The listing builds one solid part. Answer for the finished solid, in the listing's coordinates (mm). A direction names the side the tool comes from. Give positions to 0.01 mm unless a question says otherwise; leave off trailing zeros. Order: outer loops, then holes, each group sorted by start corner. A loop starts at its lowest first (then second) coordinate and runs counter-clockwise, first axis right, second up. Notation, with made-up numbers: (2, 46.5) - (41, 46.5) arc R19 cw to (41, 77.5) - close; hole circle Ø11 at (-37.75, 9.25). An arc over 180 degrees is marked (long way). Answer in a Markdown table with one row per item.
from build123d import *

# Parameters (mm, degrees)
AUFSATZ_LINEAR_AUSTRAGEN1_DEPTH = 5


with BuildPart() as part:
    # Skizze1 → Aufsatz-Linear austragen1 (new body)
    with BuildSketch(Plane.XY):
        Polygon((460.89618142, 291.663856447), (470.89618142, 291.663856447), (470.89618142, 296.663856447), (480.89618142, 296.663856447), (480.89618142, 291.663856447), (490.89618142, 291.663856447), (490.89618142, 296.663856447), (500.89618142, 296.663856447), (500.89618142, 291.663856447), (510.89618142, 291.663856447), (510.89618142, 296.663856447), (520.89618142, 296.663856447), (520.89618142, 291.663856447), (530.89618142, 291.663856447), (530.89618142, 296.663856447), (540.89618142, 296.663856447), (540.89618142, 291.663856447), (550.89618142, 291.663856447), (550.89618142, 296.663856447), (560.89618142, 296.663856447), (560.89618142, 291.663856447), (570.89618142, 291.663856447), (570.89618142, 296.663856447), (580.89618142, 296.663856447), (580.89618142, 291.663856447), (590.89618142, 291.663856447), (590.89618142, 296.663856447), (600.89618142, 296.663856447), (600.89618142, 291.663856447), (610.89618142, 291.663856447), (610.89618142, 296.663856447), (620.89618142, 296.663856447), (620.89618142, 291.663856447), (630.89618142, 291.663856447), (630.89618142, 296.663856447), (640.89618142, 296.663856447), (640.89618142, 291.663856447), (650.89618142, 291.663856447), (680.89618142, 261.663856447), (685.89618142, 261.663856447), (685.89618142, 251.663856447), (680.89618142, 251.663856447), (680.89618142, 241.663856447), (685.89618142, 241.663856447), (685.89618142, 231.663856447), (680.89618142, 231.663856447), (680.89618142, 221.663856447), (685.89618142, 221.663856447), (685.89618142, 211.663856447), (680.89618142, 211.663856447), (680.89618142, 201.663856447), (685.89618142, 201.663856447), (685.89618142, 191.663856447), (680.89618142, 191.663856447), (680.89618142, 181.663856447), (685.89618142, 181.663856447), (685.89618142, 171.663856447), (680.89618142, 171.663856447), (680.89618142, 161.663856447), (685.89618142, 161.663856447), (685.89618142, 151.663856447), (680.89618142, 151.663856447), (680.89618142, 141.663856447), (685.89618142, 141.663856447), (685.89618142, 131.663856447), (680.89618142, 131.663856447), (680.89618142, 121.663856447), (685.89618142, 121.663856447), (685.89618142, 111.663856447), (680.89618142, 111.663856447), (680.89618142, 101.663856447), (685.89618142, 101.663856447), (685.89618142, 91.663856447), (680.89618142, 91.663856447), (680.89618142, 81.663856447), (685.89618142, 81.663856447), (685.89618142, 71.663856447), (680.89618142, 71.663856447), (680.89618142, 61.663856447), (685.89618142, 61.663856447), (685.89618142, 51.663856447), (680.89618142, 51.663856447), (680.89618142, 41.663856447), (430.89618142, 41.663856447), (430.89618142, 51.663856447), (425.89618142, 51.663856447), (425.89618142, 61.663856447), (430.89618142, 61.663856447), (430.89618142, 71.663856447), (425.89618142, 71.663856447), (425.89618142, 81.663856447), (430.89618142, 81.663856447), (430.89618142, 91.663856447), (425.89618142, 91.663856447), (425.89618142, 101.663856447), (430.89618142, 101.663856447), (430.89618142, 111.663856447), (425.89618142, 111.663856447), (425.89618142, 121.663856447), (430.89618142, 121.663856447), (430.89618142, 131.663856447), (425.89618142, 131.663856447), (425.89618142, 141.663856447), (430.89618142, 141.663856447), (430.89618142, 151.663856447), (425.89618142, 151.663856447), (425.89618142, 161.663856447), (430.89618142, 161.663856447), (430.89618142, 171.663856447), (425.89618142, 171.663856447), (425.89618142, 181.663856447), (430.89618142, 181.663856447), (430.89618142, 191.663856447), (425.89618142, 191.663856447), (425.89618142, 201.663856447), (430.89618142, 201.663856447), (430.89618142, 211.663856447), (425.89618142, 211.663856447), (425.89618142, 221.663856447), (430.89618142, 221.663856447), (430.89618142, 231.663856447), (425.89618142, 231.663856447), (425.89618142, 241.663856447), (430.89618142, 241.663856447), (430.89618142, 251.663856447), (425.89618142, 251.663856447), (425.89618142, 261.663856447), (430.89618142, 261.663856447), align=None)
        Polygon((490.89618142, 260.635021844), (620.89618142, 260.635021844), (650.89618142, 230.635021844), (650.89618142, 120.635021844), (460.89618142, 120.635021844), (460.89618142, 230.635021844), align=None, mode=Mode.SUBTRACT)
    extrude(amount=AUFSATZ_LINEAR_AUSTRAGEN1_DEPTH)


solid = part.part
Item 1: Find section D-D on x = 658.5. Write down the section's boundary in (y, z).
Answer block:
| item | result |
|---|---|
| outline | (41.66, 0) - (284.06, 0) - (284.06, 5) - (41.66, 5) - close |
Item 2: Each of these flat-tipped pins is pushed along its axis until it touches: P1, Ø2.5, axis at x = 682.5, z = 3.5, coming from the +Y side; P2, Ø2, axis at x = 522.5, z = 3.5, coming from the +Y side; P3, Ø3, axis at y = 110, z = 3, coming from the +X side. Where does it stop, or does it pass through?
Answer block:
| item | result |
|---|---|
| P1 | y = 261.66 |
| P2 | y = 291.66 |
| P3 | x = 680.9 |
Item 3: Find section B-B on y = 128. Write down the section's boundary in (x, z).
Answer block:
| item | result |
|---|---|
| outline | (430.9, 0) - (460.9, 0) - (460.9, 5) - (430.9, 5) - close; (650.9, 0) - (680.9, 0) - (680.9, 5) - (650.9, 5) - close |
Item 4: Consider line 1 (X direction, y = 148, z = 2.6); line 2 (Y direction, x = 533.5, z = 3.6); line 3 (Y direction, x = 601.5, z = 2.1). Determine where each line is inside the solid, lowest interval first.
Answer block:
| item | result |
|---|---|
| line 1 | 430.9 to 460.9, 650.9 to 680.9 |
| line 2 | 41.66 to 120.64, 260.64 to 296.66 |
| line 3 | 41.66 to 120.64, 260.64 to 291.66 |
Item 5: Determine the mould class of faces 1 (the face through (558, 114, 5)), 2 (the face through (665.69, 276.87, 2.46)), 3 (the face through (475.69, 245.43, 2.46)) for opening direction X: pulls with the +X half, pulls with the -X half, needs draft (parallel to the pull), parting line crosses it, or undercut.
Answer block:
| item | result |
|---|---|
| face 1 | needs draft |
| face 2 | pulls with the +X half |
| face 3 | undercut |
Item 6: Find section C-C on y = 67.5. Write down the section's boundary in (x, z).
Answer block:
| item | result |
|---|---|
| outline | (430.9, 0) - (680.9, 0) - (680.9, 5) - (430.9, 5) - close |
Item 7: Find section A-A on x = 576.5. Write down the section's boundary in (y, z).
Answer block:
| item | result |
|---|---|
| outline | (41.66, 0) - (120.64, 0) - (120.64, 5) - (41.66, 5) - close; (260.64, 0) - (296.66, 0) - (296.66, 5) - (260.64, 5) - close |
Item 8: Which of the six approach directions +Z, -Z, +X, -X, +Y, -Y give full straight-line access (tool end or side, diameter ignored) to faces 4 (the face through (445.686, 276.454, 2.465)), 5 (the face through (635.686, 245.845, 2.465))?
Answer block:
| item | result |
|---|---|
| face 4 | +Z, -Z, -X, +Y |
| face 5 | +Z, -Z |
